For this review, use the dimensioned drawing (mm, ordinates from the lowest corner) and the shaded views. Give positions to 0.01 mm unless a question says otherwise; leave off trailing zeros. Return JSON: item names as keys, results as strings.
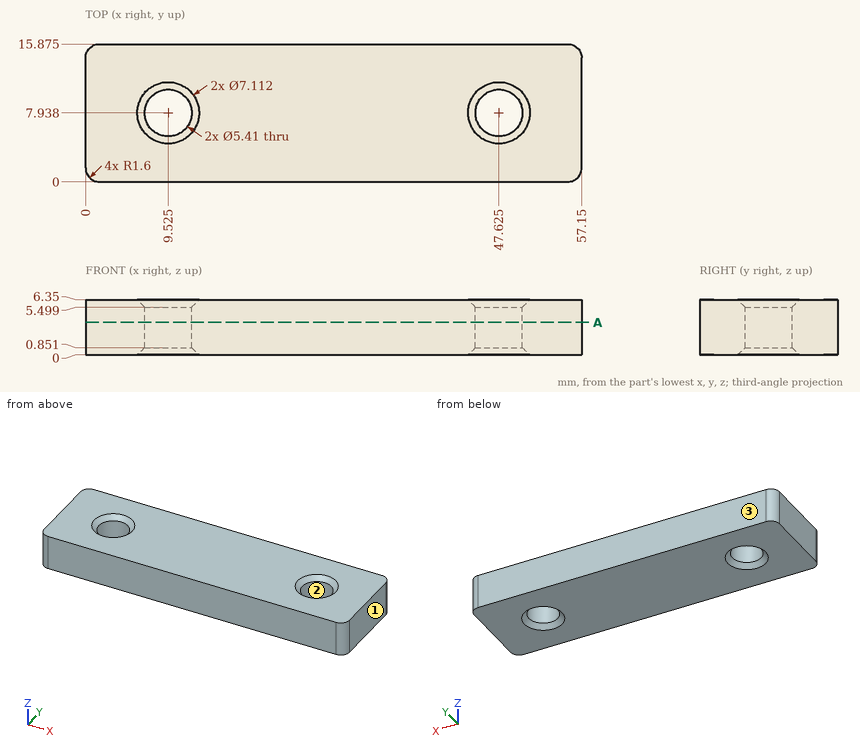
1. To check wall thickness, follow probe 1 along X at (y, z) = (8.5, 2.5); probe 2 along Y at (x, z) = (48.5, 3.25) (1 decimal); probe 3 along Y at (x, z) = (8.5, 2.75) (1 decimal). State the ranges of each line that lie inside material, in increasing order.
Results found:
{"probe 1": "x = 0 to 6.88, 12.17 to 44.98, 50.27 to 57.15", "probe 2": "y = 0 to 5.4, 10.5 to 15.9", "probe 3": "y = 0 to 5.4, 10.4 to 15.9"}
2. Add section A-A, the plane z = 3.75. Count the separate pieces of the cut face and the enclosed holes in it, plus the area to 3 significant figures.
Results found:
{"separate pieces": "1", "enclosed holes": "2", "area": "859 mm²"}
3. The part is to be moulded in two halves that separate along X. For the marked faces 1, 2 and 3, say which applies: +X half, -X half, draft (parallel to the pull), parting line (faces both ways), or undercut.
Results found:
{"face 1": "+X half", "face 2": "undercut", "face 3": "draft"}
4. For pin 1 (7 mm diameter, centred on x = 47.62, y = 7.94, fed in from -Z), flat-tipped, find the tip position at first contact; note if it passes through.
Results found:
{"pin 1": "stops at z = 0.05"}
